Model file for the job. Use its own axes, mm. A direction names the side the tool comes from. Round coordinates to 2 decimals unless told otherwise and drop trailing zeros. Loops run counter-clockwise (first coordinate to the right, second up) from the corner with the lowest first, then second, coordinate; pieces in that order, holes last. Notation, with made-up numbers: M -4,-18.5 L 18,-18.5 A25 ccw 18,4.5 Z; hole C -9,-15.5 d8. An arc over 180 degrees is marked long. Use a Markdown table: item, result. Add a question column.
Q1. Pin check, flat tips, straight feed: pin 1 (1 mm diameter, centred on x = 44, z = -9, fed in from +Y); pin 2 (2.5 mm diameter, centred on x = 69.5, z = -64.5, fed in from -Y); pin 3 (4 mm diameter, centred on x = 69.5, z = -5.5, fed in from +Y); pin 4 (2 mm diameter, centred on x = 17.75, z = -66.16, fed in from -Y). Stop position of each tip, or through.
Q2. Tool access for faces 1 (the face through (5.306, 2.986, -65.765)), 2 (the face through (59.65, 0.99, -4.24)): list every direction of +Z, -Z, +X, -X, +Y, -Y with a clear straight run to the whole face (end or side of a thin tool).
Q3. Cut at C-C (z = -13.5). Give the cut face in (x, y), plus the area to 3 significant figures.
Q4. Probe line 1 (X direction, y = 3.7, z = -27.5); line 2 (Z direction, x = 18, y = 4.85); line 3 (Z direction, x = 45.5, y = 3.2). List the from-to ranges inside material, lowest first. Write a range as from..to.
Q5. Mould opens along X. For faces 3 (the face through (0, 3, -35)), 4 (the face through (56.18, 3.73, -69.66)), 5 (the face through (36, 3, -70)) say: +X half, -X half, draft (parallel to the pull), parting line (faces both ways), or undercut.
Q6. Cut at D-D (x = 62). Give the cut face in (y, z).
Q7. Cut at B-B (x = 51). Give the cut face in (y, z), plus the area to 3 significant figures.
Q8. Cut at A-A (x = 12.5). Give the cut face in (y, z).
from build123d import *

# Parameters (mm, degrees)
SKETCH1_R           = 1.85
BOSS_EXTRUDE1_DEPTH = 2
SKETCH2_W           = 74
SKETCH2_H           = 70
SKETCH2_R           = 1.5
BOSS_EXTRUDE2_DEPTH = 2
SKETCH3_W           = 74
SKETCH3_H           = 70
BOSS_EXTRUDE3_DEPTH = 1.5


with BuildPart() as part:
    # Sketch1 → Boss-Extrude1 (new body)
    with BuildSketch(Plane(origin=(0, 0, 0), x_dir=(1, 0, 0), z_dir=(0, 1, 0))):
        Polygon((0, 0), (74, 0), (74, 70), (56.753344727, 70), (55.746655273, 70), (18.253344727, 70), (17.246655273, 70), (0, 70), align=None)
        with Locations((17.75, 66.160760925)):
            Circle(SKETCH1_R, mode=Mode.SUBTRACT)
        with Locations((12.5, 4.160760925)):
            Circle(SKETCH1_R, mode=Mode.SUBTRACT)
        with Locations((61.5, 4.160760925)):
            Circle(SKETCH1_R, mode=Mode.SUBTRACT)
        with Locations((56.25, 66.160760925)):
            Circle(SKETCH1_R, mode=Mode.SUBTRACT)
    extrude(amount=BOSS_EXTRUDE1_DEPTH)

    # Sketch2 → Boss-Extrude2 (add)
    with BuildSketch(Plane(origin=(0, 2, 0), x_dir=(1, 0, 0), z_dir=(0, 1, 0))):
        with Locations((37, 35)):
            Rectangle(SKETCH2_W, SKETCH2_H)
        with Locations((4.5, 5.5)):
            Circle(SKETCH2_R, mode=Mode.SUBTRACT)
        with Locations((69.5, 5.5)):
            Circle(SKETCH2_R, mode=Mode.SUBTRACT)
        with Locations((69.5, 64.5)):
            Circle(SKETCH2_R, mode=Mode.SUBTRACT)
        with Locations((4.5, 64.5)):
            Circle(SKETCH2_R, mode=Mode.SUBTRACT)
        with BuildLine():
            Line((4.5, 3), (9.198086301, 3))
            ThreePointArc((9.198086301, 3), (12.5, 0.660760925), (15.801913699, 3))
            Line((15.801913699, 3), (58.198086301, 3))
            ThreePointArc((58.198086301, 3), (61.5, 0.660760925), (64.801913699, 3))
            Line((64.801913699, 3), (69.5, 3))
            ThreePointArc((69.5, 3), (67.732233047, 7.267766953), (72, 5.5))
            Line((72, 5.5), (72, 64.5))
            ThreePointArc((72, 64.5), (67.732233047, 62.732233047), (69.5, 67))
            Line((69.5, 67), (59.647893138, 67))
            ThreePointArc((59.647893138, 67), (56.25, 69.660760925), (52.852106862, 67))
            Line((52.852106862, 67), (21.147893138, 67))
            ThreePointArc((21.147893138, 67), (17.75, 69.660760925), (14.352106862, 67))
            Line((14.352106862, 67), (4.5, 67))
            ThreePointArc((4.5, 67), (6.267766953, 62.732233047), (2, 64.5))
            Line((2, 64.5), (2, 5.5))
            ThreePointArc((2, 5.5), (6.267766953, 7.267766953), (4.5, 3))
        make_face(mode=Mode.SUBTRACT)
    extrude(amount=BOSS_EXTRUDE2_DEPTH)

    # Sketch3 → Boss-Extrude3 (add)
    with BuildSketch(Plane(origin=(0, 4, 0), x_dir=(1, 0, 0), z_dir=(0, 1, 0))):
        with Locations((37, 35)):
            Rectangle(SKETCH3_W, SKETCH3_H)
        with BuildLine():
            Line((9.198086301, 3), (2, 3))
            Line((2, 3), (2, 67))
            Line((2, 67), (4.5, 67))
            Line((4.5, 67), (14.352106862, 67))
            ThreePointArc((14.352106862, 67), (17.75, 69.660760925), (21.147893138, 67))
            Line((21.147893138, 67), (52.852106862, 67))
            ThreePointArc((52.852106862, 67), (56.25, 69.660760925), (59.647893138, 67))
            Line((59.647893138, 67), (72, 67))
            Line((72, 67), (72, 64.6))
            Line((72, 64.6), (72, 3))
            Line((72, 3), (64.801913699, 3))
            ThreePointArc((64.801913699, 3), (61.5, 0.660760925), (58.198086301, 3))
            Line((58.198086301, 3), (15.801913699, 3))
            ThreePointArc((15.801913699, 3), (12.5, 0.660760925), (9.198086301, 3))
        make_face(mode=Mode.SUBTRACT)
    extrude(amount=BOSS_EXTRUDE3_DEPTH)


solid = part.part
Checked values:
| question | item | result |
|---|---|---|
| 1 | pin 1 | stops at y = 2 |
| 1 | pin 2 | stops at y = 0 |
| 1 | pin 3 | stops at y = 4 |
| 1 | pin 4 | passes through |
| 2 | face 1 | +Y |
| 2 | face 2 | +Y, -Y |
| 3 | outline | M 0,0 L 74,0 L 74,5.5 L 72,5.5 L 72,2 L 2,2 L 2,5.5 L 0,5.5 Z |
| 3 | area | 162 mm^2 |
| 4 | line 1 | x = 0..2, 72..74 |
| 4 | line 2 | z = -70..-69.65, -3..0 |
| 4 | line 3 | z = -70..-67, -3..0 |
| 5 | face 3 | -X half |
| 5 | face 4 | undercut |
| 5 | face 5 | draft |
| 6 | outline | M 0,-70 L 5.5,-70 L 5.5,-67 L 2,-67 L 2,-5.94 L 0,-5.94 Z; M 0,-2.38 L 2,-2.38 L 2,-0.7 L 5.5,-0.7 L 5.5,0 L 0,0 Z |
| 7 | outline | M 0,-70 L 5.5,-70 L 5.5,-67 L 2,-67 L 2,-3 L 5.5,-3 L 5.5,0 L 0,0 Z |
| 7 | area | 161 mm^2 |
| 8 | outline | M 0,-70 L 5.5,-70 L 5.5,-67 L 2,-67 L 2,-6.01 L 0,-6.01 Z; M 0,-2.31 L 2,-2.31 L 2,-0.66 L 5.5,-0.66 L 5.5,0 L 0,0 Z |
